Read the model definition and answer for the solid it produces. Units are mm, in the model's axes. Coordinates: 2 decimals unless noted, no trailing zeros. Order: outer loops, then holes, each group sorted by start corner. A loop starts at its lowest first (then second) coordinate and runs counter-clockwise, first axis right, second up. Notation, with made-up numbers: (-26.75, 68.25) -> (25.25, 68.25) arc R24 cw to (25.25, 82.25) -> close; hole circle Ø6 at (-2.5, -39.5). An arc over 180 degrees is marked (long way). Answer in a Markdown table with one row per item.
Autodesk Inventor part; units mm, degrees
ref_plane "YZ Plane" through (0, 0, 0) normal (1, 0, 0) x (0, 1, 0)
ref_plane "XZ Plane" through (0, 0, 0) normal (0, 1, 0) x (-1, 0, 0)
ref_plane "XY Plane" through (0, 0, 0) normal (0, 0, 1) x (1, 0, 0)
sketch "Sketch1" plane through (0, 0, 0) normal (0, 0, 1) x (1, 0, 0)
  line L0 (-219.75, -149.75) -> (219.75, -149.75)
  line L1 (219.75, -149.75) -> (219.75, 149.75)
  line L2 (219.75, 149.75) -> (-219.75, 149.75)
  line L3 (-219.75, 149.75) -> (-219.75, -149.75)
  line L4 (-219.75, -149.75) -> (219.75, 149.75) construction
  line L5 (219.75, -149.75) -> (-219.75, 149.75) construction
  point P0 (0, 0)
  dimension "d0" = 439.5
  dimension "d1" = 299.5
extrude "Extrusion1" add sketch "Sketch1" along normal blind 3
fillet "Fillet1" radius 20 4 edges at (219.75, 149.75, 1.5) (219.75, -149.75, 1.5) (-219.75, -149.75, 1.5) (-219.75, 149.75, 1.5)
sketch "Sketch2" plane through (0, 0, 3) normal (0, 0, 1) x (1, 0, 0)
  line L0 (-313.799, 0) -> (313.799, 0) construction
  line L1 (-199.75, -149.75) -> (199.75, -149.75)
  arc A0 (-219.75, -129.75) -> (-199.75, -149.75) centre (-199.75, -129.75) ccw
  line L2 (-219.75, 129.75) -> (-219.75, -129.75)
  arc A1 (-199.75, 149.75) -> (-219.75, 129.75) centre (-199.75, 129.75) ccw
  line L3 (199.75, 149.75) -> (-199.75, 149.75)
  arc A2 (219.75, 129.75) -> (199.75, 149.75) centre (199.75, 129.75) ccw
  line L4 (219.75, -129.75) -> (219.75, 129.75)
  arc A3 (199.75, -149.75) -> (219.75, -129.75) centre (199.75, -129.75) ccw
  line L5 (199.75, -134.75) -> (-199.75, -134.75)
  arc A4 (-204.75, -129.75) -> (-199.75, -134.75) centre (-199.75, -129.75) ccw
  line L6 (-204.75, -129.75) -> (-204.75, 129.75)
  arc A5 (-199.75, 134.75) -> (-204.75, 129.75) centre (-199.75, 129.75) ccw
  line L7 (-199.75, 134.75) -> (199.75, 134.75)
  arc A6 (204.75, 129.75) -> (199.75, 134.75) centre (199.75, 129.75) ccw
  line L8 (204.75, 129.75) -> (204.75, -129.75)
  arc A7 (199.75, -134.75) -> (204.75, -129.75) centre (199.75, -129.75) ccw
  line L9 (204.75, 55.25) -> (165.25, 55.25)
  line L10 (165.25, 55.25) -> (165.25, -134.75)
  line L11 (165.25, -134.75) -> (204.75, -134.75)
  line L12 (204.75, -134.75) -> (204.75, 55.25)
  dimension "d7" = 15
  dimension "d8" = 370
  dimension "d9" = 190
extrude "Extrusion2" cut sketch "Sketch2" against normal through all contours L5 A4 L6 A5 L7 A6 L8 L9 L10
fillet "Fillet2" radius 7 3 edges at (204.75, 55.25, 1.5) (165.25, 55.25, 1.5) (165.25, -134.75, 1.5)
sketch "Sketch4" plane through (0, 0, 3) normal (0, 0, 1) x (1, 0, 0)
  line L0 (165.25, 48.25) -> (165.25, -127.75)
  line L1 (165.25, -124.75) -> (-206.75, -124.75)
  line L2 (-206.75, -124.75) -> (-206.75, -134.75)
  line L3 (-206.75, -134.75) -> (165.25, -134.75)
  line L4 (165.25, -134.75) -> (165.25, -124.75)
  line L5 (-206.75, 134.75) -> (204.75, 134.75)
  line L6 (204.75, 134.75) -> (204.75, 124.75)
  line L7 (204.75, 124.75) -> (-206.75, 124.75)
  line L8 (-206.75, 124.75) -> (-206.75, 134.75)
  line L9 (-199.75, 134.75) -> (199.75, 134.75)
  line L10 (158.25, -134.75) -> (-199.75, -134.75)
  point P0 (0, 0)
  point P1 (-1, 134.75)
  point P2 (204.75, 129.75)
  point P3 (-20.75, -134.75)
  point P4 (165.25, -127.75)
  dimension "d13" = 10
  dimension "d14" = 10
extrude "Extrusion3" add sketch "Sketch4" against normal up to surface (3 mm away)
fillet "Fillet3" radius 7 4 edges at (204.75, 124.75, 1.5) (-204.75, 124.75, 1.5) (-204.75, -124.75, 1.5) (165.25, -124.75, 1.5)
sketch "Sketch5" plane through (0, 0, 3) normal (0, 0, 1) x (1, 0, 0)
  line L0 (204.75, 117.75) -> (204.75, 62.25)
  arc A0 (197.75, 55.25) -> (204.75, 62.25) centre (197.75, 62.25) ccw
  line L1 (197.75, 55.25) -> (172.25, 55.25)
  arc A1 (172.25, 55.25) -> (165.25, 48.25) centre (172.25, 48.25) ccw
  line L2 (165.25, 48.25) -> (165.25, -117.75)
  arc A2 (158.25, -124.75) -> (165.25, -117.75) centre (158.25, -117.75) ccw
  line L3 (158.25, -124.75) -> (-197.75, -124.75)
  arc A3 (-204.75, -117.75) -> (-197.75, -124.75) centre (-197.75, -117.75) ccw
  line L4 (-204.75, -117.75) -> (-204.75, 117.75)
  arc A4 (-197.75, 124.75) -> (-204.75, 117.75) centre (-197.75, 117.75) ccw
  line L5 (-197.75, 124.75) -> (197.75, 124.75)
  arc A5 (204.75, 117.75) -> (197.75, 124.75) centre (197.75, 117.75) ccw
  arc A6 (-199.75, 149.75) -> (-219.75, 129.75) centre (-199.75, 129.75) ccw
  line L6 (-219.75, 129.75) -> (-219.75, -129.75)
  arc A7 (-219.75, -129.75) -> (-199.75, -149.75) centre (-199.75, -129.75) ccw
  line L7 (-199.75, -149.75) -> (199.75, -149.75)
  arc A8 (199.75, -149.75) -> (219.75, -129.75) centre (199.75, -129.75) ccw
  line L8 (219.75, -129.75) -> (219.75, 129.75)
  arc A9 (219.75, 129.75) -> (199.75, 149.75) centre (199.75, 129.75) ccw
  line L9 (199.75, 149.75) -> (-199.75, 149.75)
  point P0 (0, 0)
equation "\"d14\" = d13"
properties part number "UpperAcrylicPlate"
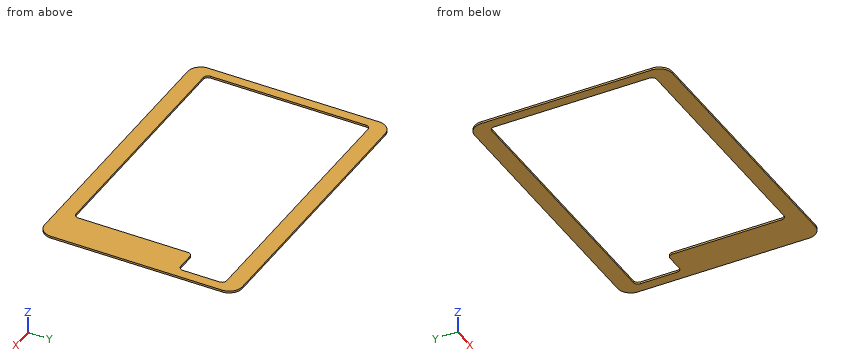
Q1. The part is cut by section B-B (y = -49.5). Write down the section's boundary in (x, z), then the cut area to 4 significant figures.
Outcome:
| item | result |
|---|---|
| outline | (-219.75, 0) -> (-204.75, 0) -> (-204.75, 3) -> (-219.75, 3) -> close; (165.25, 0) -> (219.75, 0) -> (219.75, 3) -> (165.25, 3) -> close |
| area | 208.5 mm² |
Q2. The part is cut by section C-C (z = 0.75). Write down the section's boundary in (x, y), then the cut area to 3 significant figures.
Outcome:
| item | result |
|---|---|
| outline | (-219.75, -129.75) arc R20 ccw to (-199.75, -149.75) -> (199.75, -149.75) arc R20 ccw to (219.75, -129.75) -> (219.75, 129.75) arc R20 ccw to (199.75, 149.75) -> (-199.75, 149.75) arc R20 ccw to (-219.75, 129.75) -> close; hole (-204.75, -117.75) arc R7 ccw to (-197.75, -124.75) -> (158.25, -124.75) arc R7 ccw to (165.25, -117.75) -> (165.25, 48.25) arc R7 cw to (172.25, 55.25) -> (197.75, 55.25) arc R7 ccw to (204.75, 62.25) -> (204.75, 117.75) arc R7 ccw to (197.75, 124.75) -> (-197.75, 124.75) arc R7 ccw to (-204.75, 117.75) -> close |
| area | 36,300 mm² |
Q3. Consider line 1 (X direction, y = 26.5, z = 1.35); line 2 (Y direction, x = 59, z = 0.65); line 3 (Y direction, x = 188, z = 1.7). Determine where each line is inside the solid, lowest interval first.
Outcome:
| item | result |
|---|---|
| line 1 | -219.75 to -204.75, 165.25 to 219.75 |
| line 2 | -149.75 to -124.75, 124.75 to 149.75 |
| line 3 | -149.75 to 55.25, 124.75 to 149.75 |
Q4. The part is cut by section A-A (x = -161.5). Write down the section's boundary in (y, z), then the cut area to 3 significant figures.
Outcome:
| item | result |
|---|---|
| outline | (-149.75, 0) -> (-124.75, 0) -> (-124.75, 3) -> (-149.75, 3) -> close; (124.75, 0) -> (149.75, 0) -> (149.75, 3) -> (124.75, 3) -> close |
| area | 150 mm² |
